Here's how the part is built. I have some questions about the finished solid (model axes, mm). Round coordinates to 2 decimals unless told otherwise and drop trailing zeros. Order: outer loops, then holes, each group sorted by start corner. A loop starts at its lowest first (then second) coordinate and runs counter-clockwise, first axis right, second up. Notation, with made-up numbers: (31, 38.5) - (53, 38.5) arc R25 ccw to (53, 77.5) - close; hole circle Ø1 at (16.25, -20). An arc over 180 degrees is marked (long way). One line per item, written item: value.
from build123d import *

# Parameters (mm, degrees)
ESBO_O1_W                    = 60
ESBO_O1_H                    = 45
RESSALTO_EXTRUS_O1_DEPTH     = 3
FURO_DE_DI_METRO_3_0_3_1_D   = 3
ESBO_O9_W                    = 3
ESBO_O9_H                    = 4.5
ESBO_O9_H_2                  = 2.25
CORTE_EXTRUS_O2_DEPTH        = 38.619808612
PERFIL_CORTE_W               = 23
PERFIL_CORTE_H               = 12.4
CORTE_PRINCIPAL_DEPTH        = 71.704257164
FURO_DE_DI_METRO_2_6_2_6_1_D = 2.6
FILETE1_R                    = 4
ESBO_O6_W                    = 15
ESBO_O6_H                    = 3
ESBO_O6_W_2                  = 10
CORTE_EXTRUS_O1_DEPTH        = 38.619808612


with BuildPart() as part:
    # Esboço1 → Ressalto-extrusão1 (new body)
    with BuildSketch(Plane(origin=(0, 0, 0), x_dir=(0, 0, -1), z_dir=(1, 0, 0))):
        Rectangle(ESBO_O1_W, ESBO_O1_H)
    extrude(amount=RESSALTO_EXTRUS_O1_DEPTH)

    # Furo de diâmetro Ø3.0 (3)1 (through all)
    with Locations(Plane(origin=(3, 0, 0), x_dir=(0, 0, -1), z_dir=(1, 0, 0))):
        with Locations((-25.7, -11.25), (25.7, -11.25)):
            Hole(FURO_DE_DI_METRO_3_0_3_1_D / 2)

    # Esboço9 → Corte-extrusão2 (cut, through all)
    with BuildSketch(Plane(origin=(0, 0, 0), x_dir=(0, 0, -1), z_dir=(1, 0, 0))):
        with Locations((-25.7, -18.5)):
            Rectangle(ESBO_O9_W, ESBO_O9_H)
        with Locations((-25.7, -2.875)):
            Rectangle(ESBO_O9_W, ESBO_O9_H_2)
        with Locations((-25.7, -6.625)):
            Rectangle(ESBO_O9_W, ESBO_O9_H_2)
        with Locations((25.7, -18.5)):
            Rectangle(ESBO_O9_W, ESBO_O9_H)
        with Locations((25.7, -4)):
            Rectangle(ESBO_O9_W, ESBO_O9_H)
    extrude(amount=CORTE_EXTRUS_O2_DEPTH, mode=Mode.SUBTRACT)

    # Perfil Corte → Corte Principal (cut, through all)
    with BuildSketch(Plane(origin=(3, -11.32307532, -32.016865102), x_dir=(0, 0, -1), z_dir=(1, 0, 0))):
        with Locations((-41.516865102, 21.32307532)):
            Rectangle(PERFIL_CORTE_W, PERFIL_CORTE_H)
    extrude(amount=-CORTE_PRINCIPAL_DEPTH, mode=Mode.SUBTRACT)

    # Furo de diâmetro Ø2.6 (2.6)1 (through all)
    with Locations(Plane(origin=(3, -5, 96.504216275), x_dir=(0, 0, -1), z_dir=(1, 0, 0))):
        with Locations((87.004216275, 25), (87.004216275, 5)):
            Hole(FURO_DE_DI_METRO_2_6_2_6_1_D / 2)

    # Filete1
    filete1_edges = [part.edges().sort_by_distance(p)[0] for p in [
        (1.5, 22.5, 30),
        (1.5, 22.5, -30),
        (1.5, -22.5, -30),
        (1.5, -22.5, 30),
    ]]
    fillet(filete1_edges, radius=FILETE1_R)

    # Esboço6 → Corte-extrusão1 (cut, through all)
    with BuildSketch(Plane(origin=(0, 0, 0), x_dir=(0, 0, -1), z_dir=(1, 0, 0))):
        with Locations((-14.8, -16.25)):
            Rectangle(ESBO_O6_W, ESBO_O6_H)
        with Locations((17.7, -16.25)):
            Rectangle(ESBO_O6_W_2, ESBO_O6_H)
    extrude(amount=CORTE_EXTRUS_O1_DEPTH, mode=Mode.SUBTRACT)


solid = part.part
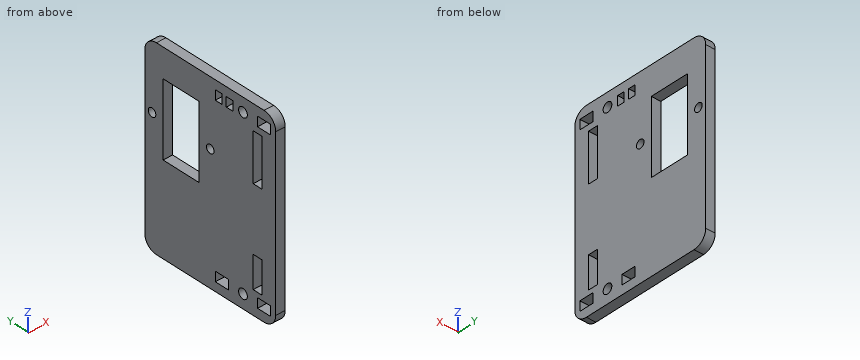
Q1. If we section it at D-D, the plane y = -10.5: Please give me the cut outline in (x, z), then the cut area to 3 significant figures.
Results list:
outline: (0, -30) - (3, -30) - (3, -27) - (0, -27) - close; (0, -24.4) - (3, -24.4) - (3, 24.4) - (0, 24.4) - close; (0, 27) - (3, 27) - (3, 30) - (0, 30) - close
area: 164 mm²
Q2. If we section it at B-B, the plane y = 8: Please give me the cut outline in (x, z), then the cut area to 3 significant figures.
Results list:
outline: (0, -30) - (3, -30) - (3, -2) - (0, -2) - close; (0, 21) - (3, 21) - (3, 30) - (0, 30) - close
area: 111 mm²
Q3. If we section it at C-C, the plane z = 13: Please give me the cut outline in (x, y), then the cut area to 3 significant figures.
Results list:
outline: (0, -22.5) - (3, -22.5) - (3, -17.75) - (0, -17.75) - close; (0, -14.75) - (3, -14.75) - (3, 3.8) - (0, 3.8) - close; (0, 16.2) - (3, 16.2) - (3, 22.5) - (0, 22.5) - close
area: 88.8 mm²
Q4. Will this pin go through, and if not, where does the flat tip stop? pin 1 (1.6 mm diameter, centred on y = 0, z = 9.5, fed in from +X).
Results list:
pin 1: through
Q5. If we section it at A-A, the plane z = -1: Please give me the cut outline in (x, y).
Results list:
outline: (0, -22.5) - (3, -22.5) - (3, 3.8) - (0, 3.8) - close; (0, 16.2) - (3, 16.2) - (3, 22.5) - (0, 22.5) - close
Q6. If I drill on line 1 along Y through (x, z) = (1.1, 16); line 2 along Y through (x, z) = (1.75, 25.7); line 3 along Y through (x, z) = (1.3, -25.7), over which ranges is the centre line in solid material (lowest first)?
Results list:
line 1: -22.5 to -17.75, -14.75 to 3.8, 16.2 to 22.5
line 2: -22.5 to -20.75, -16.25 to -12.75, -9.75 to -7.75, -5.5 to -4, -1.75 to 22.5
line 3: -22.5 to -20.75, -16.25 to -12.75, -9.75 to -6.25, -1.75 to 22.5
